```python
from build123d import *

# Parameters (mm, degrees)
F3_DEPTH  = 3.302
F4_R      = 4.826
F5_DEPTH  = 6.35
F6_R      = 25.4
F7_DEPTH  = 76.2
F8_R      = 44.45
F9_DEPTH  = 6.35
F10_R     = 3.81
F11_DEPTH = 25.4


with BuildPart() as f1:
    # F0 (on Front) → F1 (revolve)
    with BuildSketch(Plane.XZ):
        Polygon((0, 59.4741), (0, 0), (12.7, 0), (12.7, 50.8), (5.626218, 50.8), (3.302, 59.4741), align=None)
    revolve(axis=Axis((-7.589792, 0, 0), (1, 0, 0)))

    # F2 (on Right) → F3 (cut)
    with BuildSketch(Plane.YZ):
        with BuildLine():
            Line((4.826, -62.648721), (4.826, 38.1))
            ThreePointArc((4.826, 38.1), (0, 42.926), (-4.826, 38.1))
            Line((-4.826, 38.1), (-4.826, -62.648721))
            Line((-4.826, -62.648721), (4.826, -62.648721))
        make_face()
    extrude(amount=F3_DEPTH, mode=Mode.SUBTRACT)

    # F4 (on Right) → F5 (cut)
    with BuildSketch(Plane.YZ):
        with Locations((0, 38.1)):
            Circle(F4_R)
    extrude(amount=F5_DEPTH, mode=Mode.SUBTRACT)

    # F6 (on face) → F7 (join)
    with BuildSketch(Plane.YZ.offset(12.7)):
        Circle(F6_R)
    extrude(amount=F7_DEPTH)

    # F8 (on face) → F9 (join)
    with BuildSketch(Plane.YZ.offset(88.9)):
        Circle(F8_R)
    extrude(amount=F9_DEPTH)

    # F10 (on face) → F11 (cut)
    with BuildSketch(Plane.YZ.offset(95.25)):
        with Locations((-36.5125, 0)):
            Circle(F10_R)
        with Locations((18.25625, -31.620753)):
            Circle(F10_R)
        with Locations((18.25625, 31.620753)):
            Circle(F10_R)
    extrude(amount=-F11_DEPTH, mode=Mode.SUBTRACT)


solid = f1.part
```
The model under review builds one solid part; all positions refer to its coordinate system, in mm. A direction names the side the tool comes from. Round coordinates to 2 decimals unless told otherwise and drop trailing zeros. Loops run counter-clockwise (first coordinate to the right, second up) from the corner with the lowest first, then second, coordinate; pieces in that order, holes last. Notation, with made-up numbers: (80.25, 45) -> (133.25, 45) arc R18 cw to (133.25, 61) -> close; hole circle Ø8 at (-32.75, -26.5). An arc over 180 degrees is marked (long way). Answer as a JSON object with one key per item and string values. Group by question number.
1) For pin 1 Ø9 at (y, z) = (-36.51, 0) entering from -X; pin 2 Ø8 at (x, z) = (47, -22.5) entering from +Y; pin 3 Ø5 at (y, z) = (-0.5, 37.5) entering from -X; pin 4 Ø8 at (y, z) = (41.5, 36.5) entering from +X, all flat-tipped, find the tip position at first contact; note any pin that passes through.
2) Mouldability with a two-part tool opening along X and no side actions: class faces 1 (the face through (50.267, -5.506, -24.796)), 2 (the face through (3.836, -0.628, 42.885)), 3 (the face through (0, 12, -1)) as released by +X, released by -X, zero draft, split by the parting line, or undercut.
3) For faces 4 (the face through (12.7, -23.3, -10.6)), 5 (the face through (6.35, 0, 38)), 6 (the face through (2, 4.826, -11)), 7 (the face through (92.031, 42.397, 13.352)), list the 3-axis set-ups (+Z, -Z, +X, -X, +Y, -Y) from which the entire face can be reached by the end or side of a thin tool; tool diameter is ignored.
4) We need section B-B on y = -37.5. Give the number of separate pieces and of enclosed holes in the cut face, then the cut area to 3 significant figures.
5) We need section C-C on x = 70.5. Write out the cut boundary in (y, z), then the cut area to 3 significant figures.
6) For line 1 (X direction, y = 41, z = 11.5); line 2 (X direction, y = -42.5, z = 26); line 3 (Z direction, x = 62.5, y = -6.5), list the stretches that pass through material, from the lowest coordinate up. Write a range as [from, to].
7) We need section A-A on z = 0. Write out the cut boundary in (x, y), then the cut area to 3 significant figures.
Result set:
{
 "1": {"pin 1": "x = 0", "pin 2": "y = 17.4", "pin 3": "x = 6.35", "pin 4": "x = 5.5"},
 "2": {"face 1": "undercut", "face 2": "zero draft", "face 3": "released by -X"},
 "3": {"face 4": "none", "face 5": "-X", "face 6": "-Z, -X", "face 7": "+X"},
 "4": {"separate pieces": "3", "enclosed holes": "0", "area": "1,230 mm²"},
 "5": {"outline": "circle Ø50.8 at (0, 0)", "area": "2,030 mm²"},
 "6": {"line 1": "[0, 12.7], [88.9, 95.25]", "line 2": "[0, 12.7]", "line 3": "[-24.55, 24.55]"},
 "7": {"outline": "(0, -59.47) -> (3.3, -59.47) -> (5.63, -50.8) -> (12.7, -50.8) -> (12.7, -25.4) -> (88.9, -25.4) -> (88.9, -32.7) -> (95.25, -32.7) -> (95.25, 44.45) -> (88.9, 44.45) -> (88.9, 25.4) -> (12.7, 25.4) -> (12.7, 50.8) -> (5.63, 50.8) -> (3.3, 59.47) -> (0, 59.47) -> (0, 4.83) -> (3.3, 4.83) -> (3.3, -4.83) -> (0, -4.83) -> close; (88.9, -44.45) -> (95.25, -44.45) -> (95.25, -40.32) -> (88.9, -40.32) -> close", "area": "5,720 mm²"}
}
